```python
from build123d import *

# Parameters (mm, degrees)
SKETCH1_R           = 2.1
BOSS_EXTRUDE1_DEPTH = 5
SKETCH3_W           = 30
SKETCH3_H           = 5
BOSS_EXTRUDE2_DEPTH = 15
SKETCH4_R           = 2.6
CUT_EXTRUDE2_DEPTH  = 108.425323176
FILLET2_R           = 10
SKETCH5_R           = 4.4
CUT_EXTRUDE3_DEPTH  = 108.425323272
SKETCH2_R           = 3.6
CUT_EXTRUDE4_DEPTH  = 114.974558916
BOSS_EXTRUDE3_DEPTH = 25
FILLET3_R           = 5
SKETCH7_R           = 2.1
CUT_EXTRUDE5_DEPTH  = 114.974558956


with BuildPart() as part:
    # Sketch1 → Boss-Extrude1 (new body)
    with BuildSketch(Plane.XY):
        Polygon((73.634936481, -21), (73.634936481, -20), (103.634936481, -20), (103.634936481, -21), (103.634936481, -45), (73.634936481, -45), align=None)
        with Locations((98.634936481, -35.1)):
            Circle(SKETCH1_R, mode=Mode.SUBTRACT)
        with Locations((78.634936481, -35.1)):
            Circle(SKETCH1_R, mode=Mode.SUBTRACT)
        with Locations((98.634936481, -25.1)):
            Circle(SKETCH1_R, mode=Mode.SUBTRACT)
        with Locations((78.634936481, -25.1)):
            Circle(SKETCH1_R, mode=Mode.SUBTRACT)
    extrude(amount=BOSS_EXTRUDE1_DEPTH)

    # Sketch3 → Boss-Extrude2 (add)
    with BuildSketch(Plane.XY.offset(5)):
        with Locations((88.634936481, -42.5)):
            Rectangle(SKETCH3_W, SKETCH3_H)
    extrude(amount=BOSS_EXTRUDE2_DEPTH)

    # Sketch4 → Cut-Extrude2 (cut, through all)
    with BuildSketch(Plane(origin=(0, -40, 0), x_dir=(1, 0, 0), z_dir=(0, 1, 0))):
        with Locations(Location((88.634936481, -12.5, 0), (0, 0, 180))):
            Circle(SKETCH4_R)
    extrude(amount=-CUT_EXTRUDE2_DEPTH, mode=Mode.SUBTRACT)

    # Fillet2
    # the kernel refuses this fillet: 10 mm, written as the material it adds along each edge
    with BuildSketch(Plane(origin=(73.634936481, -40, 5), x_dir=(0, 0, 1), z_dir=(1, 0, 0))) as fillet2_piece_1_section:
        with BuildLine():
            CenterArc((FILLET2_R, -FILLET2_R), FILLET2_R, 90, 90)
            Line((0, -FILLET2_R), (0, 0))
            Line((0, 0), (FILLET2_R, 0))
        make_face()
    fillet2_piece_1 = extrude(amount=30, mode=Mode.PRIVATE)
    fillet2_piece_1 = fillet2_piece_1 - Plane(origin=(88.634936481, -37.846712749, 12.5), x_dir=(-1, 0, 0), z_dir=(0, 1, 0)) * Cylinder(2.6, 100, mode=Mode.PRIVATE)
    fillet2_piece_1 = fillet2_piece_1 - Plane(origin=(98.634936481, -35.1, 7.280393082), x_dir=(1, 0, 0), z_dir=(0, 0, -1)) * Cylinder(2.1, 100, mode=Mode.PRIVATE)
    fillet2_piece_1 = fillet2_piece_1 - Plane(origin=(78.634936481, -35.1, 7.280393082), x_dir=(1, 0, 0), z_dir=(0, 0, -1)) * Cylinder(2.1, 100, mode=Mode.PRIVATE)
    add(fillet2_piece_1)

    # Sketch5 → Cut-Extrude3 (cut, through all)
    with BuildSketch(Plane(origin=(0, -40, 0), x_dir=(1, 0, 0), z_dir=(0, 1, 0))):
        with Locations((88.634936481, -12.5)):
            Circle(SKETCH5_R)
    extrude(amount=CUT_EXTRUDE3_DEPTH, mode=Mode.SUBTRACT)

    # Sketch2 → Cut-Extrude4 (cut, through all)
    with BuildSketch(Plane.XY.offset(5)):
        with Locations((98.634936481, -25.1)):
            Circle(SKETCH2_R)
        with Locations(Location((98.634936481, -35.1, 0), (0, 0, 180))):
            Circle(SKETCH2_R)
        with Locations((78.634936481, -25.1)):
            Circle(SKETCH2_R)
        with Locations(Location((78.634936481, -35.1, 0), (0, 0, 180))):
            Circle(SKETCH2_R)
    extrude(amount=CUT_EXTRUDE4_DEPTH, mode=Mode.SUBTRACT)

    # Sketch6 → Boss-Extrude3 (add)
    with BuildSketch(Plane.XZ.offset(45)):
        with BuildLine():
            Line((88.634936481, 0), (73.634936481, 0))
            Line((73.634936481, 0), (73.634936481, -2.430609057))
            ThreePointArc((73.634936481, -2.430609057), (81.037110141, -0.611589546), (88.634936481, 0))
        make_face()
        with BuildLine():
            Line((103.634936481, 0), (88.634936481, 0))
            ThreePointArc((88.634936481, 0), (96.232762821, -0.611589546), (103.634936481, -2.430609057))
            Line((103.634936481, -2.430609057), (103.634936481, 0))
        make_face()
    extrude(amount=-BOSS_EXTRUDE3_DEPTH)

    # Fillet3
    fillet3_edges = [part.edges().sort_by_distance(p)[0] for p in [
        (103.634936481, -20, 1.284695471),
        (73.634936481, -20, 1.284695471),
    ]]
    fillet(fillet3_edges, radius=FILLET3_R)

    # Sketch7 → Cut-Extrude5 (cut, through all)
    with BuildSketch(Plane.XY.offset(5)):
        with Locations((98.634936481, -35.1)):
            Circle(SKETCH7_R)
        with Locations((98.634936481, -25.1)):
            Circle(SKETCH7_R)
        with Locations((78.634936481, -25.1)):
            Circle(SKETCH7_R)
        with Locations((78.634936481, -35.1)):
            Circle(SKETCH7_R)
    extrude(amount=-CUT_EXTRUDE5_DEPTH, mode=Mode.SUBTRACT)


solid = part.part
```
Could you check a few things on this model? Use its own coordinates, in mm. A direction names the side the tool comes from. Round coordinates to 2 decimals unless told otherwise and drop trailing zeros. Write each loop counter-clockwise with the first axis right and the second up, starting at its lowest first coordinate (ties: lowest second). Pieces come first, ordered by that corner, then holes. Notation, with made-up numbers: M 75,37.5 L 103,37.5 A17 ccw 103,61.5 Z; hole C -8,-14.5 d8. An arc over 180 degrees is marked long. Write each question's results on one line, items separated by ' | '. Start each with the question number.
1. Thinking about a two-plate mould opening in Z: for faces 1 (the face through (73.635, -37, 6)), 2 (the face through (88, -36, 7)), 3 (the face through (87.44, -42.46, 10.19)), which applies, +Z half, -Z half, draft (parallel to the pull), parting line (faces both ways), or undercut?
2. On a 3-axis mill with a long thin cutter (end or side, diameter ignored), from which of +Z, -Z, +X, -X, +Y, -Y can I reach the whole of each face in a straight line? I mean faces 4 (the face through (89, -25, 5)), 5 (the face through (75.138, -21.426, 1.233)), 6 (the face through (79.1, -38.67, 6.94)). Say none if no direction works.
3. I need wall thicknesses on L1, parallel to X at y = -35.1, z = -1.2; L2, parallel to X at y = -43.15, z = 12.5; L3, parallel to Y at x = 80.5, z = -0.5. Which ranges of each line are inside material? Lowest first, please. Write a range as from..to.
4. Imagine slicing it at D-D on y = -35.1. List the corners of the cut face in (x, z) for me, and give its area (3 significant figures).
5. Imagine slicing it at A-A on x = 77.5. List the corners of the cut face in (y, z) for me, and give its area (3 significant figures).
6. Imagine slicing it at C-C on x = 86.5. List the corners of the cut face in (y, z) for me, and give its area (3 significant figures).
7. I'm going to push flat-ended pins straight in: pin 1 Ø6.5 at (x, y) = (98.63, -25.1) entering from +Z; pin 2 Ø4 at (y, z) = (-30.5, 6.5) entering from -X; pin 3 Ø9.5 at (x, y) = (98.63, -35.1) entering from -Z; pin 4 Ø7 at (x, z) = (88.63, 12.5) entering from +Y. Where does each tip first touch, or does it pass through?
Result sheet:
1) face 1: draft | face 2: +Z half | face 3: undercut
2) face 4: +Z, +X, -X, +Y | face 5: +Z, -Z, -X, +Y | face 6: +Z
3) L1: x = 73.63..76.53, 100.73..103.63 | L2: x = 73.63..86.03, 91.23..103.63 | L3: y = -45..-36.07, -34.13..-26.07, -24.13..-20
4) outline: M 73.63,-2.43 A47.5 cw 76.53,-1.57 L 76.53,5 L 75.03,5 L 75.03,6.4 L 73.63,6.4 Z; M 80.73,-0.66 A47.5 cw 96.53,-0.66 L 96.53,5 L 95.03,5 L 95.03,6.4 L 82.23,6.4 L 82.23,5 L 80.73,5 Z; M 100.73,-1.57 A47.5 cw 103.63,-2.43 L 103.63,6.4 L 102.23,6.4 L 102.23,5 L 100.73,5 Z | area: 145 mm^2
5) outline: M -45,-1.32 L -36.87,-1.32 L -36.87,5 L -38.52,5 L -38.52,9.76 A10 cw -40,15 L -40,20 L -45,20 Z; M -33.33,-1.32 L -26.87,-1.32 L -26.87,5 L -30,5 A10 cw -31.68,5.14 L -31.68,5 L -33.33,5 Z; M -23.33,-1.32 L -20.13,-1.32 L -20.13,5 L -23.33,5 Z | area: 197 mm^2
6) outline: M -45,-0.05 L -20,-0.05 L -20,5 L -30,5 A10 cw -37.73,8.65 L -40,8.65 L -40,11.02 L -45,11.02 Z; M -45,13.98 L -40,13.98 L -40,20 L -45,20 Z | area: 203 mm^2
7) pin 1: stops at z = 5 | pin 2: stops at x = 73.63 | pin 3: stops at z = -2.35 | pin 4: stops at y = -40
